Autodesk Inventor part; units mm, degrees
ref_plane "YZ Plane" through (0, 0, 0) normal (1, 0, 0) x (0, 1, 0)
ref_plane "XZ Plane" through (0, 0, 0) normal (0, 1, 0) x (-1, 0, 0)
ref_plane "XY Plane" through (0, 0, 0) normal (0, 0, 1) x (1, 0, 0)
sketch "Sketch1" plane through (0, 0, 0) normal (0, 0, 1) x (1, 0, 0)
  line L0 (-30.1, 0) -> (30.1, 0) construction
  line L1 (0, 42) -> (0, -42) construction
  line L2 (-21.5, -30) -> (21.5, -30)
  line L3 (21.5, -30) -> (21.5, 30)
  line L4 (21.5, 30) -> (-21.5, 30)
  line L5 (-21.5, 30) -> (-21.5, -30)
  line L6 (-21.5, -30) -> (21.5, 30) construction
  line L7 (21.5, -30) -> (-21.5, 30) construction
  point P0 (0, 0)
  dimension "d0" = 43
  dimension "d1" = 60
extrude "Extrusion1" add sketch "Sketch1" along normal blind 300
sketch "Sketch4" plane through (-21.5, -30, 0) normal (-1, 0, 0) x (0, 0, 1)
  line L0 (0, 60) -> (0, 0) construction
  line L1 (-60, 30) -> (360, 30) construction
  line L2 (0, 38) -> (5, 38)
  line L3 (13, 30) -> (13, 30)
  line L4 (5, 22) -> (0, 22)
  line L5 (0, 22) -> (0, 38)
  arc A0 (13, 30) -> (5, 38) centre (5, 30) ccw
  arc A1 (5, 22) -> (13, 30) centre (5, 30) ccw
  point P0 (0, 30)
  point P1 (13, 22)
  point P2 (13, 38)
  dimension "d7" = 16
  dimension "d8" = 13
  dimension "d9" = 8
extrude "Extrusion3" cut sketch "Sketch4" against normal through all
sketch "Sketch5" plane through (0, 0, 0) normal (0, 0, -1) x (-1, 0, 0)
  line L0 (0, -42) -> (0, 42) construction
  line L1 (-30.1, 0) -> (30.1, 0) construction
  line L2 (-10.75, -19) -> (10.75, -19) construction
  line L3 (10.75, -19) -> (10.75, 19) construction
  line L4 (10.75, 19) -> (-10.75, 19) construction
  line L5 (-10.75, 19) -> (-10.75, -19) construction
  line L6 (-10.75, -19) -> (10.75, 19) construction
  line L7 (10.75, -19) -> (-10.75, 19) construction
  line L8 (21.5, -30) -> (-21.5, -30)
  line L9 (-21.5, 30) -> (21.5, 30)
  line L10 (21.5, -8) -> (-21.5, -8) construction
  line L11 (-21.5, 8) -> (21.5, 8) construction
  point P0 (0, 0)
  dimension "d12" = 21.5
  dimension "d13" = 38
  dimension "d14" = 60
  dimension "d15" = 16
  dimension "d16" = 43
hole "Hole1" at (10.75, 19, 0) at (-10.75, 19, 0) at (-10.75, -19, 0) at (10.75, -19, 0) direction (0, 0, 1) diameter 4.134 depth 14.2 tip angle 118 countersink diameter 5 countersink angle 90
equation "\"d9\" = 0.5 * d7"
equation "\"d12\" = 0.5 * d16"
equation "\"d13\" = 0.5 * d14 + 0.5 * d15"
properties part number "10-002-ARM" material "Aluminum 6061"
For this review, take the finished solid that the model builds, in its own axes (mm). A direction names the side the tool comes from. Round coordinates to 2 decimals unless told otherwise and drop trailing zeros. Write each loop counter-clockwise with the first axis right and the second up, starting at its lowest first coordinate (ties: lowest second). Pieces come first, ordered by that corner, then holes. Notation, with made-up numbers: M -36.5,8.5 L -21.5,8.5 A24 cw -21.5,45.5 Z; hole C -7,56 d10. An arc over 180 degrees is marked long. One line per item, written item: value. Start each with the question number.
(1) Wall thickness on line 1 (X direction, y = 19, z = 4.25); line 2 (Y direction, x = -10.75, z = 8.75); line 3 (Y direction, x = 10, z = 5): over which ranges is each line inside the solid? List them lowest first.
(2) We need section A-A (y = 0). Give the boundary of the cut face in (x, z), and give its area (3 significant figures).
(3) Machinability: for faces 4 (the flat face through (-21.5, 0, 148)), 5 (the flat face through (0, -8, 3)), which of the approach directions +Z, -Z, +X, -X, +Y, -Y give a long, thin tool a straight path to every point of the face, cutting with its end or side? Answer none if there is none.
(4) The part is to be moulded in two halves that separate along Y. For faces 1 (the flat face through (0, 8, 2)), 2 (the flat face through (0, -30, 148)), 3 (the flat face through (0, 0, 300)), say which applies: released by +Y, released by -Y, zero draft, split by the parting line, or undercut.
Result:
1. line 1: -21.5 to -12.82, -8.68 to 8.68, 12.82 to 21.5
1. line 2: -30 to -21.07, -16.93 to -7.07, 7.07 to 16.93, 21.07 to 30
1. line 3: -30 to -20.93, -17.07 to -8, 8 to 17.07, 20.93 to 30
2. outline: M -21.5,13 L 21.5,13 L 21.5,300 L -21.5,300 Z
2. area: 12,300 mm²
3. face 4: +Z, -Z, -X, +Y, -Y
3. face 5: -Z, +X, -X
4. face 1: undercut
4. face 2: released by -Y
4. face 3: zero draft
